from build123d import *

# Parameters (mm, degrees)
BOSS_EXTRUDE1_DEPTH                    = 6.35
SKETCH3_W                              = 8.466666667
SKETCH3_H                              = 8.466666667
SKETCH3_W_2                            = 8.466666666
BOSS_EXTRUDE2_DEPTH                    = 6.349999915
SKETCH8_W                              = 8.466666666
SKETCH8_H                              = 8.466666666
BOSS_EXTRUDE4_DEPTH                    = 19.049999915
CUT_EXTRUDE1_DEPTH                     = 5.08
CUT_EXTRUDE2_DEPTH                     = 5.08
CUT_EXTRUDE3_DEPTH                     = 5.08
CHAMFER1_SIZE                          = 0.635
SKETCH7_R                              = 8
BOSS_EXTRUDE3_DEPTH                    = 4.233333333
CHAMFER2_SIZE                          = 2.116666709
CUT_EXTRUDE5_DEPTH                     = 2.54
F_18_0_1695_DIAMETER_HOLE1_D           = 4.3053
F_18_0_1695_DIAMETER_HOLE1_DEPTH       = 4.572
F_18_0_1695_DIAMETER_HOLE1_CSINK_D     = 5.5753
F_18_0_1695_DIAMETER_HOLE1_CSINK_ANGLE = 90
F_18_0_1695_DIAMETER_HOLE1_TIP         = 1.293442612


with BuildPart() as part:
    # Sketch2 → Boss-Extrude1 (new body)
    with BuildSketch(Plane(origin=(0, 0, 0), x_dir=(1, 0, 0), z_dir=(0, 1, 0))):
        Polygon((93.233827842, 63.000000026), (93.233827842, -71.466666693), (-84.767161176, -71.466666693), (-84.767161176, -63.000000026), (84.767161176, -63.000000026), (84.767161176, 63.000000026), align=None)
    extrude(amount=BOSS_EXTRUDE1_DEPTH)

    # Sketch3 → Boss-Extrude2 (add)
    with BuildSketch(Plane(origin=(0, 6.35, 0), x_dir=(1, 0, 0), z_dir=(0, 1, 0))):
        with Locations((-80.533827843, -67.23333336)):
            Rectangle(SKETCH3_W, SKETCH3_H)
        with Locations((89.000494509, -67.23333336)):
            Rectangle(SKETCH3_W_2, SKETCH3_H)
    extrude(amount=BOSS_EXTRUDE2_DEPTH)

    # Sketch8 → Boss-Extrude4 (add)
    with BuildSketch(Plane(origin=(0, 6.35, 0), x_dir=(1, 0, 0), z_dir=(0, 1, 0))):
        with Locations((89.000494509, 58.766666693)):
            Rectangle(SKETCH8_W, SKETCH8_H)
    extrude(amount=BOSS_EXTRUDE4_DEPTH)

    # Sketch4 → Cut-Extrude1 (cut)
    with BuildSketch(Plane.ZY.offset(84.767161176)):
        Polygon((64.05833336, 8.466666667), (67.23333336, 11.641666667), (70.40833336, 8.466666667), (67.23333336, 5.291666667), align=None)
    extrude(amount=-CUT_EXTRUDE1_DEPTH, mode=Mode.SUBTRACT)

    # Sketch5 → Cut-Extrude2 (cut)
    with BuildSketch(Plane(origin=(0, 0, -63.000000026), x_dir=(-1, 0, 0), z_dir=(0, 0, -1))):
        Polygon((-92.175494509, 8.466666667), (-89.000494509, 11.641666667), (-85.825494509, 8.466666667), (-89.000494509, 5.291666667), align=None)
        Polygon((-92.175494509, 21.166666582), (-89.000494509, 24.341666582), (-85.825494509, 21.166666582), (-89.000494509, 17.991666582), align=None)
    extrude(amount=-CUT_EXTRUDE2_DEPTH, mode=Mode.SUBTRACT)

    # Sketch6 → Cut-Extrude3 (cut)
    with BuildSketch(Plane.XZ):
        Polygon((85.825494509, 67.23333336), (89.000494509, 70.40833336), (92.175494509, 67.23333336), (89.000494509, 64.05833336), align=None)
    extrude(amount=-CUT_EXTRUDE3_DEPTH, mode=Mode.SUBTRACT)

    # Chamfer1
    chamfer1_edges = [part.edges().sort_by_distance(p)[0] for p in [
        (87.412994509, 5.08, 65.64583336),
        (87.412994509, 5.08, 68.82083336),
        (90.587994509, 5.08, 68.82083336),
        (90.587994509, 5.08, 65.64583336),
        (87.412994509, 0, 65.64583336),
        (90.587994509, 0, 65.64583336),
        (90.587994509, 0, 68.82083336),
        (87.412994509, 0, 68.82083336),
        (-79.687161176, 6.879166667, 65.64583336),
        (-79.687161176, 10.054166667, 65.64583336),
        (-79.687161176, 10.054166667, 68.82083336),
        (-79.687161176, 6.879166667, 68.82083336),
        (-84.767161176, 6.879166667, 65.64583336),
        (-84.767161176, 6.879166667, 68.82083336),
        (-84.767161176, 10.054166667, 68.82083336),
        (-84.767161176, 10.054166667, 65.64583336),
        (90.587994509, 6.879166667, -57.920000026),
        (90.587994509, 10.054166667, -57.920000026),
        (87.412994509, 10.054166667, -57.920000026),
        (87.412994509, 6.879166667, -57.920000026),
        (90.587994509, 6.879166667, -63.000000026),
        (87.412994509, 6.879166667, -63.000000026),
        (87.412994509, 10.054166667, -63.000000026),
        (90.587994509, 10.054166667, -63.000000026),
        (90.587994509, 19.579166582, -57.920000026),
        (90.587994509, 22.754166582, -57.920000026),
        (87.412994509, 22.754166582, -57.920000026),
        (87.412994509, 19.579166582, -57.920000026),
        (90.587994509, 19.579166582, -63.000000026),
        (87.412994509, 19.579166582, -63.000000026),
        (87.412994509, 22.754166582, -63.000000026),
        (90.587994509, 22.754166582, -63.000000026),
    ]]
    chamfer(chamfer1_edges, length=CHAMFER1_SIZE)

    # Sketch7 → Boss-Extrude3 (add)
    with BuildSketch(Plane(origin=(93.233827842, 0, 0), x_dir=(0, 0, -1), z_dir=(1, 0, 0))):
        with BuildLine():
            Line((20.666666693, 25.399999915), (20.666666693, 6.35))
            Line((20.666666693, 6.35), (54.53333336, 6.35))
            Line((54.53333336, 6.35), (54.53333336, 25.399999915))
            Line((54.53333336, 25.399999915), (63.000000026, 25.399999915))
            ThreePointArc((63.000000026, 25.399999915), (41.83333336, 46.566666582), (20.666666693, 25.399999915))
        make_face()
        with Locations((41.83333336, 25.399999915)):
            Circle(SKETCH7_R, mode=Mode.SUBTRACT)
    extrude(amount=-BOSS_EXTRUDE3_DEPTH)

    # Chamfer2
    chamfer2_edges = [part.edges().sort_by_distance(p)[0] for p in [
        (-76.300494509, 12.699999915, 67.23333336),
        (86.883827842, 25.399999915, -54.53333336),
        (89.000494509, 12.699999915, 63.000000026),
        (93.233827842, 12.699999915, 67.23333336),
        (89.000494509, 12.699999915, 71.466666693),
        (84.767161176, 12.699999915, 67.23333336),
    ]]
    chamfer(chamfer2_edges, length=CHAMFER2_SIZE)

    # Sketch9 → Cut-Extrude5 (cut)
    with BuildSketch(Plane(origin=(0, 6.35, 0), x_dir=(1, 0, 0), z_dir=(0, 1, 0))):
        with BuildLine():
            Line((-76.300494509, -67.233333526), (-76.300494509, -63.000000026))
            Line((-76.300494509, -63.000000026), (-68.426494509, -63.000000026))
            Line((-68.426494509, -63.000000026), (-68.426494509, -67.233333526))
            ThreePointArc((-68.426494509, -67.233333526), (-72.363494509, -71.170333526), (-76.300494509, -67.233333526))
        make_face()
        with BuildLine():
            Line((89.000494676, -55.126000026), (84.767161176, -55.126000026))
            Line((84.767161176, -55.126000026), (84.767161176, -63.000000026))
            Line((84.767161176, -63.000000026), (89.000494676, -63.000000026))
            ThreePointArc((89.000494676, -63.000000026), (92.937494676, -59.063000026), (89.000494676, -55.126000026))
        make_face()
    extrude(amount=-CUT_EXTRUDE5_DEPTH, mode=Mode.SUBTRACT)

    # #18 (0.1695) Diameter Hole1
    with Locations(Plane(origin=(0, 3.81, 0), x_dir=(1, 0, 0), z_dir=(0, 1, 0))):
        with Locations((89.000494676, -59.063000026), (-72.363494509, -67.233333526)):
            CounterSinkHole(F_18_0_1695_DIAMETER_HOLE1_D / 2, F_18_0_1695_DIAMETER_HOLE1_CSINK_D / 2, depth=F_18_0_1695_DIAMETER_HOLE1_DEPTH, counter_sink_angle=F_18_0_1695_DIAMETER_HOLE1_CSINK_ANGLE)
            with Locations((0, 0, -(F_18_0_1695_DIAMETER_HOLE1_DEPTH + F_18_0_1695_DIAMETER_HOLE1_TIP / 2))):  # 118° drill point
                Cone(0, F_18_0_1695_DIAMETER_HOLE1_D / 2, F_18_0_1695_DIAMETER_HOLE1_TIP, mode=Mode.SUBTRACT)


solid = part.part
Verification items for the finished model (mm, model axes). A direction names the side the tool comes from. Coordinates: 2 decimals unless noted, no trailing zeros. Order: outer loops, then holes, each group sorted by start corner. A loop starts at its lowest first (then second) coordinate and runs counter-clockwise, first axis right, second up.
Item 1: Material ranges on L1, parallel to X at y = 32, z = -46.5; L2, parallel to Z at x = -19, y = 4.5; L3, parallel to Y at x = 82.5, z = 66.5, recorded low to high.
Filled in:
L1: x = 89 to 93.23
L2: z = 63 to 71.47
L3: y = 0 to 6.35
Item 2: Section check A-A, the plane z = -47. Enter the section's corners in (x, y), then the cut area to 3 significant figures.
Filled in:
outline: (84.77, 0) - (93.23, 0) - (93.23, 19.29) - (89, 19.29) - (89, 6.35) - (84.77, 6.35) - close; (89, 31.51) - (93.23, 31.51) - (93.23, 45.93) - (89, 45.93) - close
area: 170 mm2
Item 3: Depth check by flat-ended pin: pin 1 (3.5 mm diameter, centred on x = -72.36, z = 67.23, fed in from +Y); pin 2 (2 mm diameter, centred on y = 8.5, z = 66, fed in from -X); pin 3 (8.5 mm diameter, centred on x = 87.5, z = 59, fed in from +Y); pin 4 (12 mm diameter, centred on x = 11, y = 8.5, fed in from -Z). Enter the tip coordinate at first touch or a pass-through.
Filled in:
pin 1: passes through
pin 2: stops at x = -79.97
pin 3: stops at y = 10.83
pin 4: stops at z = 63
Item 4: Section check D-D, the plane z = 3. Enter the section's corners in (x, y), then the cut area to 3 significant figures.
Filled in:
outline: (84.77, 0) - (93.23, 0) - (93.23, 6.35) - (84.77, 6.35) - close
area: 53.8 mm2
Item 5: Section check B-B, the plane y = 28.5. Enter the section's corners in (x, z), then the cut area to 3 significant figures.
Filled in:
outline: (89, -62.77) - (93.23, -62.77) - (93.23, -49.21) - (89, -49.21) - close; (89, -34.46) - (93.23, -34.46) - (93.23, -20.89) - (89, -20.89) - close
area: 115 mm2
Item 6: Section check C-C, the plane x = -23.5. Enter the section's corners in (y, z).
Filled in:
outline: (0, 63) - (6.35, 63) - (6.35, 71.47) - (0, 71.47) - close
Item 7: Access from +Z, -Z, +X, -X, +Y, -Y to the whole of each face (thin tool, end or side, straight path). Record for faces 4 (the face through (90.84, 0.32, 65.45)), 5 (the face through (90.84, 10.25, -62.68)), 6 (the face through (84.767, 6, -9)), 7 (the face through (-84.445, 10.304, 69.014)).
Filled in:
face 4: -Y
face 5: -Z
face 6: -Z, -X, +Y, -Y
face 7: -X
Item 8: Release check for a two-part mould opening along X. For faces 1 (the face through (89, 6.35, 3)), 2 (the face through (93.234, 15, -25)), 3 (the face through (87.16, 6.69, -62.68)) record: +X half, -X half, draft (parallel to the pull), parting line (faces both ways), or undercut.
Filled in:
face 1: draft
face 2: +X half
face 3: undercut
